Autodesk Fusion 360 part; units mm, degrees
sketch "Sketch1" plane through (0, 0, 0) normal (0, 1, 0) x (1, 0, 0)
  line L0 (0, -3.2) -> (-3, -3.2)
  line L1 (-3, -3.2) -> (-3, -3)
  line L2 (-3, -3) -> (-1.5, -1.5)
  line L3 (-1.5, -1.5) -> (-1.5, 4.8)
  line L4 (-1.5, -1.5) -> (0, 0) construction
  line L5 (-1.5, 4.8) -> (0, 4.8)
  line L6 (0, 4.8) -> (0, -3.2)
  dimension "d5" = 45
  dimension "d9" = 3
  dimension "d10" = 8
  dimension "d72" = 1.7
  dimension "d73" = 6
revolve "Revolve1" add sketch "Sketch1" angle 360 about axis through (0, 0, -4.8) along (0, 0, 1)
sketch "Sketch6" plane through (0, 0, 3.2) normal (0, 0, 1) x (1, 0, 0)
  circle A0 centre (0, 0) radius 3
  line L0 (-1, 0) -> (1, 0) construction
  line L1 (-1, -0.5774) -> (-1, 0.5774)
  line L2 (-1, 0.5774) -> (0, 0)
  line L3 (-1, -0.5774) -> (0, 0)
  dimension "d65" = 2
  dimension "d67" = 60
extrude "Extrude1" cut sketch "Sketch6" against normal blind 1.2 contours L1 L2 L3
pattern_circular "C-Pattern1" count 6 over 360 about axis through (0, 0, 1.75) along (0, 0, 1) of "Extrude1"
extrude "Extrude2" cut 1 faces at (-0.3333, 0.1925, 2) along direction (0, 0, -1) blind 1.2
fillet "Fillet6" radius 0.1 1 edges at (-1.3985, 0.5424, 1.5)
thread "Thread2" thread offset 0 thread length 5.3
sketch "Sketch8" plane through (0, 0, 0) normal (0, 1, 0) x (1, 0, 0)
  line L0 (-3, -3.2) -> (-3, -3)
  line L1 (-3, -3) -> (-1.5, -1.5)
  line L2 (0, 4.8) -> (0, -3.2)
  line L3 (0, -3.2) -> (-3, -3.2)
  line L4 (0, 4.8) -> (-1.53, 4.8)
  line L5 (-1.53, 4.8) -> (-1.53, 4.5)
  line L6 (-1.53, 4.5) -> (-1.2, 4.8)
  dimension "d104" = 1.2
  dimension "d106" = 1.53
  dimension "d107" = 0.3
revolve "Revolve3" cut sketch "Sketch8" angle 360 about axis through (0, 0, -4.8) along (0, 0, 1)
equation "d5 = adsk_headang * 0.5"
equation "d9 = adsk_nomdia"
equation "d10 = adsk_nomlen"
equation "adsk_nomlen = 8.00 mm"
equation "adsk_headh = 1.70 mm"
equation "adsk_headdia = 6.00 mm"
equation "adsk_nomdia = 3.00 mm"
equation "adsk_headang = 90.00 deg"
equation "adsk_philwidth = 2.00 mm"
equation "adsk_phildepth = 1.20 mm"
equation "d65 = adsk_philwidth"
equation "d72 = adsk_headh"
equation "d73 = adsk_headdia"
equation "d77 = adsk_thrlen"
equation "adsk_thrlen = 5.30 mm"
equation "adsk_midfillet = 0.10 mm"
equation "d85 = adsk_midfillet"
equation "adsk_startlen = adsk_nomdia * 0.1"
equation "d99 = ( adsk_nomdia / 2 ) * tan(90 deg - adsk_headang / 2) + adsk_headh"
equation "adsk_endpointdia = adsk_nomdia - 2 * adsk_startlen"
equation "d104 = adsk_endpointdia / 2"
equation "d106 = adsk_nomdia * 0.51"
equation "d107 = adsk_startlen"
properties part number "arrangementsContainer"
Could you check a few things on this model? Use its own coordinates, in mm. A direction names the side the tool comes from. Coordinates: 2 decimals unless noted, no trailing zeros. Order: outer loops, then holes, each group sorted by start corner. A loop starts at its lowest first (then second) coordinate and runs counter-clockwise, first axis right, second up. Notation, with made-up numbers: M 77.5,67.25 L 121.5,67.25 A25 cw 121.5,104.25 Z; hole C -18,-3 d2. An arc over 180 degrees is marked long. Use one line per item in the form item = value. Start each with the question number.
1. Please list where these lines run through material, in increasing order: line 1 (Z direction, x = 0.5, y = 0); line 2 (X direction, y = -0.25, z = 1); line 3 (Z direction, x = -1, y = 2.25).
2. Suppose I cut it at A-A on z = 1. Write out the boundary of the cut face in (x, y), then the cut area to 3 significant figures.
3. We'd pull the mould along X, two halves only. Please class faces 1 (the conical face through (0, 2, 2)), 2 (the flat face through (0, 0, -4.8)), 3 (the flat face through (-1, 0, 2)): +X half, -X half, draft (parallel to the pull), parting line (faces both ways), or undercut.
4. Suppose I cut it at B-B on z = -4. Write out the boundary of the cut face in (x, y), then the cut area to 3 significant figures.
5. On a 3-axis mill with a long thin cutter (end or side, diameter ignored), from which of +Z, -Z, +X, -X, +Y, -Y can I reach the whole of each face in a straight line? I mean faces 4 (the flat face through (0.49, 0.87, 2.02)), 5 (the cylindrical face through (1.5, 0.07, -1.58)), 6 (the flat face through (-1.3, 0, 3.2)). Say none if no direction works.
6. For pin 1 (0.9 mm diameter, centred on y = 0, z = 2.5, fed in from +X); pin 2 (0.6 mm diameter, centred on x = -0.5, y = 0, fed in from +Z); pin 3 (1.5 mm diameter, centred on x = -0.5, z = -3, fed in from -Y), each with a flat end and sliding along its axis, tell me the tip position at first contact or that it passes through.
Geometry says:
q1.line_1 = -4.8 to 0.8
q1.line_2 = -1.48 to -1, 1 to 1.48
q1.line_3 = 2.46 to 3.2
q2.outline = C 0,0 d3; hole M -1,-0.58 L 0,-1.15 L 1,-0.58 L 1,0.58 L 0,1.15 L -1,0.58 Z
q2.area = 3.60 mm^2
q3.face_1 = parting line
q3.face_2 = draft
q3.face_3 = undercut
q4.outline = C 0,0 d3
q4.area = 7.07 mm^2
q5.face_4 = +Z
q5.face_5 = -Z
q5.face_6 = +Z, +X, -X, +Y, -Y
q6.pin_1 = 2.95
q6.pin_2 = 0.8
q6.pin_3 = -1.5
